from build123d import *

# Parameters (mm, degrees)
F1_DEPTH = 0.508
F2_DEPTH = 0.2032
F3_R     = 0.762
F5_R     = 1.6807405663
F6_DEPTH = 0.508
F7_D     = 2.54
F7_DEPTH = 0.509
F8_D     = 2.54
F8_DEPTH = 0.2042
F9_R     = 0.1839630735


with BuildPart() as f1:
    # F0 (on Top) → F1 (new body)
    with BuildSketch(Plane.XY):
        Polygon((-12.694504112, 12.6988124102), (-12.694504112, 6.3494062051), (-11.9335213676, 6.3494062051), (-11.9335213676, 11.9331842288), (-6.347252056, 11.9331842288), (-6.347252056, 12.6988124102), align=None)
        Polygon((-0.7515071775, 6.3494062051), (0, 6.3494062051), (0, 12.6988124102), (-6.347252056, 12.6988124102), (-6.347252056, 11.9331842288), (-0.7515071775, 11.9331842288), align=None)
        Polygon((-6.347252056, 0), (0, 0), (0, 6.3494062051), (-0.7515071775, 6.3494062051), (-0.7515071775, 0.7721490692), (-6.347252056, 0.7721490692), align=None)
        Polygon((-12.694504112, 0), (-6.347252056, 0), (-6.347252056, 0.7721490692), (-11.9335213676, 0.7721490692), (-11.9335213676, 6.3494062051), (-12.694504112, 6.3494062051), align=None)
    extrude(amount=F1_DEPTH)

    # F0 (on Top) → F2 (join)
    with BuildSketch(Plane.XY):
        Polygon((-11.9335213676, 0.7721490692), (-6.347252056, 0.7721490692), (-0.7515071775, 0.7721490692), (-0.7515071775, 6.3494062051), (-0.7515071775, 11.9331842288), (-6.347252056, 11.9331842288), (-11.9335213676, 11.9331842288), (-11.9335213676, 6.3494062051), align=None)
        Polygon((-12.694504112, 12.6988124102), (-12.694504112, 6.3494062051), (-11.9335213676, 6.3494062051), (-11.9335213676, 11.9331842288), (-6.347252056, 11.9331842288), (-6.347252056, 12.6988124102), align=None)
        Polygon((-12.694504112, 0), (-6.347252056, 0), (-6.347252056, 0.7721490692), (-11.9335213676, 0.7721490692), (-11.9335213676, 6.3494062051), (-12.694504112, 6.3494062051), align=None)
        Polygon((-6.347252056, 0), (0, 0), (0, 6.3494062051), (-0.7515071775, 6.3494062051), (-0.7515071775, 0.7721490692), (-6.347252056, 0.7721490692), align=None)
        Polygon((-0.7515071775, 6.3494062051), (0, 6.3494062051), (0, 12.6988124102), (-6.347252056, 12.6988124102), (-6.347252056, 11.9331842288), (-0.7515071775, 11.9331842288), align=None)
    extrude(amount=-F2_DEPTH)

    # F3
    f3_edges = [f1.edges().sort_by_distance(p)[0] for p in [
        (0, 0, 0.1524),
        (0, 12.698812, 0.1524),
        (-12.694504, 12.698812, 0.1524),
        (-12.694504, 0, 0.1524),
        (-11.933521, 11.933184, 0.254),
        (-11.933521, 0.772149, 0.254),
        (-0.751507, 11.933184, 0.254),
        (-0.751507, 0.772149, 0.254),
    ]]
    fillet(f3_edges, radius=F3_R)

    # F5 (on offset) → F6 (join)
    with BuildSketch(Plane.XY):
        with Locations((-6.3472064212, 6.3493414782)):
            Circle(F5_R)
    extrude(amount=F6_DEPTH)

    # F7 (through all, one way)
    with BuildSketch(Plane(origin=(0, 0, 0), x_dir=(1, 0, 0), z_dir=(0, 0, -1))):
        with Locations((-6.3472064212, -6.3493414782)):
            Circle(F7_D / 2)
    extrude(amount=-F7_DEPTH, mode=Mode.SUBTRACT)

    # F8 (through all, one way)
    with BuildSketch(Plane.XY):
        with Locations((-6.347252056, 6.3494062051)):
            Circle(F8_D / 2)
    extrude(amount=-F8_DEPTH, mode=Mode.SUBTRACT)

    # F9
    f9_edges = [f1.edges().sort_by_distance(p)[0] for p in [
        (-8.027947, 6.349341, 0.508),
        (0, 6.349406, 0.508),
        (-0.751507, 6.352667, 0.508),
        (-12.694504, 6.349406, 0.508),
        (-12.471319, 12.475628, 0.508),
        (-12.471319, 0.223185, 0.508),
        (-6.347252, 12.698812, 0.508),
        (-6.347252, 0, 0.508),
        (-0.223185, 12.475628, 0.508),
        (-0.223185, 0.223185, 0.508),
        (-6.342514, 11.933184, 0.508),
        (-11.710337, 11.71, 0.508),
        (-0.974692, 11.71, 0.508),
        (-11.933521, 6.352667, 0.508),
        (-11.710337, 0.995334, 0.508),
        (-0.974692, 0.995334, 0.508),
        (-6.342514, 0.772149, 0.508),
        (-7.617206, 6.349341, 0.508),
    ]]
    fillet(f9_edges, radius=F9_R)


solid = f1.part
Geometry: final body of the model. Coordinates: model frame, mm. A direction names the side the tool comes from. Coordinates: 2 decimals unless noted, no trailing zeros. Loops run counter-clockwise (first coordinate to the right, second up) from the corner with the lowest first, then second, coordinate; pieces in that order, holes last. Notation, with made-up numbers: (21.5, -4.5) - (79.5, -4.5) arc R10 cw to (79.5, 1.5) - close; hole circle Ø10 at (53.25, 71.25). An arc over 180 degrees is marked (long way). Put each result on its own line as item: value. Start each with the question number.
Q1. Pull-direction query (X, two-part tool) for faces 3 (the flat face through (-8, 8, 0)), 4 (the flat face through (-6.4, 12.3, 0.508)); classes: released by +X, released by -X, zero draft, split by the parting line, or undercut.
Q2. Cut plane B-B, the plane y = 4.5. Return loops of the section in (x, z).
Q3. Line query: line 1 (X direction, y = 10.25, z = 0.1); line 2 (Y direction, x = -8.5, z = 0.1); line 3 (X direction, y = 1.75, z = 0.35). Output: solid intervals per line, ascending.
Q4. Cut plane C-C, the plane x = -11. Return loops of the section in (y, z).
Q5. Set-up query: faces 1 (the flat face through (-8, 6, -0.203)), 2 (the cylindrical face through (-6.566, 8.016, 0.16)). Return all of +Z, -Z, +X, -X, +Y, -Y with unobstructed straight access to the full face (end or side cutting, diameter ignored); none if empty.
Q6. Cut plane A-A, the plane z = 0.2. Return loops of the section in (x, y), and give its area (3 significant figures).
Filled sheet:
1. face 3: undercut
1. face 4: zero draft
2. outline: (-12.69, -0.2) - (0, -0.2) - (0, 0.32) arc R0.18 ccw to (-0.18, 0.51) - (-0.57, 0.51) arc R0.18 ccw to (-0.75, 0.32) - (-0.75, 0) - (-11.93, 0) - (-11.93, 0.32) arc R0.18 ccw to (-12.12, 0.51) - (-12.51, 0.51) arc R0.18 ccw to (-12.69, 0.32) - close
3. line 1: -12.69 to -11.93, -0.75 to 0
3. line 2: 0 to 0.77, 11.93 to 12.7
3. line 3: -12.69 to -11.94, -0.75 to 0
4. outline: (0, -0.2) - (12.7, -0.2) - (12.7, 0.32) arc R0.18 ccw to (12.51, 0.51) - (12.12, 0.51) arc R0.18 ccw to (11.93, 0.32) - (11.93, 0) - (0.77, 0) - (0.77, 0.32) arc R0.18 ccw to (0.59, 0.51) - (0.18, 0.51) arc R0.18 ccw to (0, 0.32) - close
5. face 1: -Z, +X, -X, +Y, -Y
5. face 2: +Z
6. outline: (-12.69, 0.76) arc R0.76 ccw to (-11.93, 0) - (-0.76, 0) arc R0.76 ccw to (0, 0.76) - (0, 11.94) arc R0.76 ccw to (-0.76, 12.7) - (-11.93, 12.7) arc R0.76 ccw to (-12.69, 11.94) - close; circle Ø3.36 at (-6.35, 6.35); hole (-11.93, 1.53) arc R0.76 ccw to (-11.17, 0.77) - (-1.51, 0.77) arc R0.76 ccw to (-0.75, 1.53) - (-0.75, 11.17) arc R0.76 ccw to (-1.51, 11.93) - (-11.17, 11.93) arc R0.76 ccw to (-11.93, 11.17) - close; hole circle Ø2.54 at (-6.35, 6.35)
6. area: 40.2 mm²
